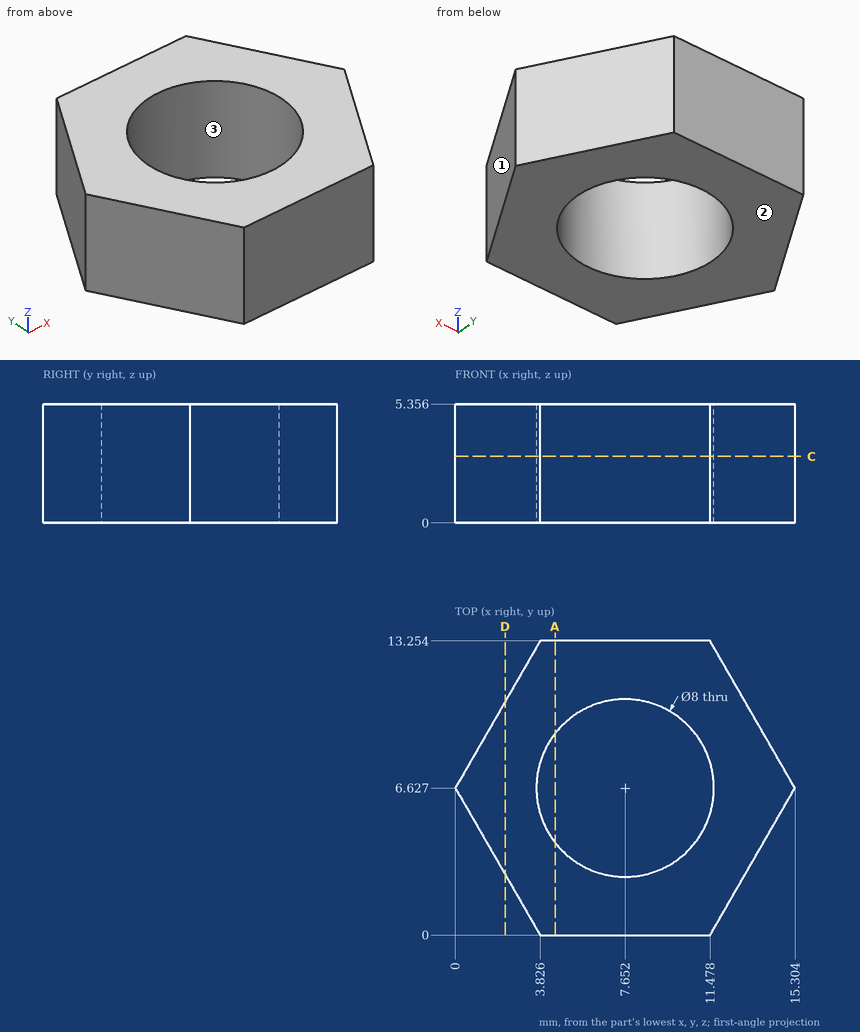
Can you work these out from the drawing? Everything is in mm from the part's minimum corner. Give positions to 0.01 mm unless a question says otherwise; leave off trailing zeros. Order: outer loops, then holes, each group sorted by start corner. A loop starts at its lowest first (then second) coordinate and runs counter-clockwise, first axis right, second up. Notation, with made-up numbers: M 47,60 L 89,60 A10 cw 89,70 Z; hole C -0.5,-14 d10. An arc over 180 degrees is marked long. Write item = value, one per line. Start each with the question number.
Q1. Suppose I cut it at C-C (z = 3). Write out the boundary of the cut face in (x, y), plus the area to 3 significant figures.
Q2. We'd pull the mould along Y, two halves only. Please class the marked faces 1, 2 and 3: pulls with the +Y half, pulls with the -Y half, needs draft (parallel to the pull), parting line crosses it, or undercut.
Q3. I need wall thicknesses on probe 1 along Y at (x, z) = (7.5, 0.35); probe 2 along X at (y, z) = (6, 4.65); probe 3 along X at (y, z) = (8.5, 2.45) (1 decimal). Which ranges of each line are inside material? Lowest first, please. Write a range as [from, to].
Q4. Suppose I cut it at D-D (x = 2.25). Write out the boundary of the cut face in (y, z).
Q5. Suppose I cut it at A-A (x = 4.5). Write out the boundary of the cut face in (y, z).
Q6. Will these pins go through, and if not, where does the flat tip stop? pin 1 Ø2 at (y, z) = (3, 3.5) entering from +X; pin 2 Ø3 at (x, y) = (13, 11) entering from -Z; pin 3 Ø5 at (x, y) = (7.65, 6.63) entering from -Z.
Check result:
q1.outline = M 0,6.63 L 3.83,0 L 11.48,0 L 15.3,6.63 L 11.48,13.25 L 3.83,13.25 Z; hole C 7.65,6.63 d8
q1.area = 102 mm2
q2.face_1 = pulls with the -Y half
q2.face_2 = needs draft
q2.face_3 = undercut
q3.probe_1 = [0, 2.63], [10.62, 13.25]
q3.probe_2 = [0.36, 3.7], [11.6, 14.94]
q3.probe_3 = [1.1, 4.1], [11.2, 14.2]
q4.outline = M 2.73,0 L 10.52,0 L 10.52,5.36 L 2.73,5.36 Z
q5.outline = M 0,0 L 4.16,0 L 4.16,5.36 L 0,5.36 Z; M 9.09,0 L 13.25,0 L 13.25,5.36 L 9.09,5.36 Z
q6.pin_1 = 13.79
q6.pin_2 = 0
q6.pin_3 = through
